Autodesk Inventor part; units mm, degrees
ref_plane "YZ Plane" through (0, 0, 0) normal (1, 0, 0) x (0, 1, 0)
ref_plane "XZ Plane" through (0, 0, 0) normal (0, 1, 0) x (-1, 0, 0)
ref_plane "XY Plane" through (0, 0, 0) normal (0, 0, 1) x (1, 0, 0)
sketch "Sketch1" plane through (0, 0, 0) normal (0, 1, 0) x (-1, 0, 0)
  line L0 (-97.5, -62.5) -> (97.5, -62.5)
  line L1 (97.5, 62.5) -> (-97.5, 62.5)
  line L2 (-97.5, 62.5) -> (-97.5, -62.5)
  line L3 (-97.5, -62.5) -> (97.5, 62.5) construction
  line L4 (97.5, -62.5) -> (-97.5, 62.5) construction
  line L5 (97.5, 20) -> (112.525, 20)
  line L6 (127.475, 21.2237) -> (127.475, -18.7763)
  line L7 (112.525, -17.5526) -> (97.5, -17.5526)
  line L8 (97.5, -62.5) -> (97.5, -17.5526)
  line L9 (97.5, 20) -> (97.5, 62.5)
  line L10 (112.525, 20) -> (112.525, 61)
  line L11 (127.475, 61) -> (127.475, 21.2237)
  line L12 (127.475, 1.2237) -> (97.475, 1.2237) construction
  line L13 (112.525, -17.5526) -> (112.525, -58.5526)
  line L14 (127.475, -58.5526) -> (127.475, -18.7763)
  line L15 (119.975, 61) -> (121.775, 61) construction
  line L16 (112.525, 61) -> (118.225, 61)
  line L17 (127.475, 61) -> (121.775, 61)
  line L18 (119.975, -58.5526) -> (121.775, -58.5526) construction
  line L19 (112.525, -58.5526) -> (118.225, -58.5526)
  line L20 (127.475, -58.5526) -> (121.775, -58.5526)
  line L21 (119.975, -58.5526) -> (121.775, -58.5526) construction
  line L22 (121.775, -58.5526) -> (121.775, -56.5526)
  line L23 (118.225, -58.5526) -> (118.225, -56.5526)
  line L24 (121.775, -56.5526) -> (125.775, -56.5526)
  line L25 (125.775, -56.5526) -> (125.775, -53.5526)
  line L26 (114.175, -53.5526) -> (118.175, -53.5526)
  line L27 (114.175, -56.5526) -> (114.175, -53.5526)
  line L28 (118.225, -56.5526) -> (114.175, -56.5526)
  line L29 (112.525, -58.5526) -> (118.225, -58.5526)
  line L30 (127.475, -58.5526) -> (121.775, -58.5526)
  line L31 (127.475, 61) -> (127.475, 79) construction
  line L32 (-97.5, 0) -> (-67.5, 0) construction
  line L33 (-67.5, 62.5) -> (-67.5, -62.5) construction
  line L34 (127.475, 79) -> (-67.5, 0) construction
  line L35 (127.475, -58.5526) -> (127.475, -76.5526) construction
  line L36 (127.475, -76.5526) -> (-67.5, 0) construction
  line L37 (-97.5, 62.5) -> (-117.5, 62.5)
  line L38 (-117.5, 62.5) -> (-117.5, -62.5)
  line L39 (-117.5, -62.5) -> (-97.5, -62.5)
  line L40 (-97.5, -62.5) -> (-97.5, 62.5)
  line L41 (-67.5, 0) -> (-47.5, 0) construction
  circle A0 centre (-47.5, 0) radius 1.6
  line L42 (-67.5, 0) -> (-87.5, 0) construction
  circle A1 centre (-87.5, 0) radius 1.6
  line L43 (121.775, 61) -> (118.225, 61)
  line L44 (125.775, -53.5526) -> (118.175, -53.5526)
  line L45 (121.775, -58.5526) -> (118.225, -58.5526)
  point P0 (0, 0)
  point P1 (-97.5, -62.5)
  dimension "d0" = 195
  dimension "d1" = 125
  dimension "d3" = 30
  dimension "d4" = 40
  dimension "d5" = 15
  dimension "d6" = 41
  dimension "d12" = 1.8
  dimension "d21" = 30
  dimension "d23" = 1.5
  dimension "d28" = 18
  dimension "d29" = 30
  dimension "d30" = 18
  dimension "d35" = 20
  dimension "d36" = 125
  dimension "d41" = 20
  dimension "d42" = 3.2
  dimension "d43" = 20
  dimension "d47" = 3.2
extrude "Extrusion1" add sketch "Sketch1" along normal blind 3.25 contours L2 L1 L9 L5 L10 L16 L43 L17 L11 L6 L14 L20 L22 L24 L25 L44 L26 L27 L28 L23 L19 L13 L7 L8 L0 | L23 L28 L27 L26 L44 L25 L24 L22 L45 | A0 | A1
sketch "Sketch2" plane through (0, 3.25, 0) normal (0, 1, 0) x (1, 0, 0)
  line L0 (-127.475, 58.5526) -> (-127.475, -61) construction
  line L1 (-127.475, 0) -> (-59.475, 0) construction
  circle A0 centre (-59.475, 0) radius 5
  point P0 (0, 0)
  dimension "d31" = 68
  dimension "d32" = 10
extrude "Extrusion2" cut sketch "Sketch2" against normal blind 10
sketch "Sketch3" plane through (97.5, 0, 62.5) normal (1, 0, 0) x (0, 0, -1)
  line L0 (125, 0) -> (80.0526, 0)
  line L1 (0, 3.25) -> (125, 3.25)
  line L2 (125, 3.25) -> (125, 0)
  line L3 (125, 0) -> (0, 0)
  line L4 (0, 0) -> (0, 3.25)
  point P0 (62.5, 0)
extrude "Extrusion4" add sketch "Sketch3" along normal blind 30
extrude "Extrusion5" cut sketch "Sketch1" along normal blind 4 contours A0 | A1
sketch "Sketch4" plane through (0, 3.25, 0) normal (0, 1, 0) x (1, 0, 0)
  line L0 (-97.5, -62.5) -> (127.5, -62.5) construction
  line L1 (39.3, -62.5) -> (39.3, -44.9) construction
  line L2 (127.5, 62.5) -> (127.5, -62.5) construction
  circle A0 centre (39.3, -44.9) radius 1.6
  circle A1 centre (16.42, -44.9) radius 1.6
  line L3 (39.3, -44.9) -> (16.42, -44.9) construction
  line L4 (118.8, -62.5) -> (118.8, -12.2) construction
  circle A2 centre (118.8, -12.2) radius 1.6
  line L5 (118.8, -12.2) -> (95.92, -12.2) construction
  circle A3 centre (95.92, -12.2) radius 1.6
  line L6 (-97.5, 62.5) -> (127.5, 62.5) construction
  line L7 (119.5, 62.5) -> (119.5, 35.9) construction
  circle A4 centre (119.5, 35.9) radius 1.6
  line L8 (119.5, 35.9) -> (96.62, 35.9) construction
  circle A5 centre (96.62, 35.9) radius 1.6
  line L9 (38.32, 62.5) -> (38.32, 33.4) construction
  circle A6 centre (38.32, 33.4) radius 1.6
  line L10 (38.32, 33.4) -> (15.44, 33.4) construction
  circle A7 centre (15.44, 33.4) radius 1.6
  point P0 (0, 0)
  point P1 (119.5, 49.2)
  dimension "d48" = 88.2
  dimension "d49" = 17.6
  dimension "d50" = 3.2
  dimension "d51" = 3.2
  dimension "d52" = 22.88
  dimension "d53" = 50.3
  dimension "d54" = 8.7
  dimension "d55" = 3.2
  dimension "d56" = 3.2
  dimension "d57" = 22.88
  dimension "d58" = 8
  dimension "d59" = 26.6
  dimension "d60" = 3.2
  dimension "d61" = 22.88
  dimension "d62" = 3.2
  dimension "d63" = 89.18
  dimension "d64" = 29.1
  dimension "d65" = 3.2
  dimension "d66" = 22.88
  dimension "d67" = 3.2
extrude "Extrusion6" cut sketch "Sketch4" against normal blind 10
sketch "Sketch5" plane through (0, 3.25, 0) normal (0, 1, 0) x (1, 0, 0)
  circle A0 centre (119.5, 35.9) radius 1.6 construction
  line L0 (123.5, 48.9829) -> (78.5, 48.9829) construction
  line L1 (123.5, 46.1029) -> (33.5, 46.1029)
  line L2 (33.5, 46.1029) -> (33.5, 51.8629)
  line L3 (33.5, 51.8629) -> (123.5, 51.8629)
  line L4 (123.5, 51.8629) -> (123.5, 46.1029)
  line L5 (123.5, 46.1029) -> (33.5, 51.8629) construction
  line L6 (33.5, 46.1029) -> (123.5, 51.8629) construction
  line L7 (127.5, 62.5) -> (127.5, -62.5)
  circle A1 centre (15.44, 33.4) radius 1.6 construction
  line L8 (11.5, 20.4) -> (56.5, 20.4) construction
  line L9 (101.5, 17.525) -> (11.5, 17.525)
  line L10 (11.5, 17.525) -> (11.5, 23.275)
  line L11 (11.5, 23.275) -> (101.5, 23.275)
  line L12 (101.5, 23.275) -> (101.5, 17.525)
  line L13 (101.5, 17.525) -> (11.5, 23.275) construction
  line L14 (11.5, 17.525) -> (101.5, 23.275) construction
  circle A2 centre (95.92, -12.2) radius 1.6 construction
  line L15 (111.5, -28.5) -> (66.5, -28.5) construction
  line L16 (124, -35.5) -> (9, -35.5)
  line L17 (9, -35.5) -> (9, -21.5)
  line L18 (9, -21.5) -> (124, -21.5)
  line L19 (124, -21.5) -> (124, -35.5)
  line L20 (124, -35.5) -> (9, -21.5) construction
  line L21 (9, -35.5) -> (124, -21.5) construction
  line L22 (-97.5, -62.5) -> (127.5, -62.5)
  point P0 (0, 0)
  dimension "d71" = 45
  dimension "d72" = 90
  dimension "d73" = 5.76
  dimension "d76" = 4
  dimension "d78" = 45
  dimension "d79" = 90
  dimension "d80" = 5.75
  dimension "d82" = 26
  dimension "d84" = 45
  dimension "d85" = 115
  dimension "d86" = 14
  dimension "d87" = 3.5
  dimension "d88" = 27
extrude "Extrusion7" cut sketch "Sketch5" against normal blind 10
sketch "Sketch8" plane through (0, 3.25, 0) normal (0, 1, 0) x (1, 0, 0)
  line L0 (-127.475, -61) -> (-112.525, -61) construction
  line L1 (-120, -61) -> (-121.75, -61) construction
  line L2 (-120, -61) -> (-118.25, -61) construction
  line L3 (-121.75, -61) -> (-121.75, -54)
  line L4 (-121.75, -54) -> (-123.95, -54)
  line L5 (-123.95, -54) -> (-123.95, -51.4)
  line L6 (-123.95, -51.4) -> (-121.75, -51.4)
  line L7 (-121.75, -51.4) -> (-121.75, -47)
  line L8 (-121.75, -47) -> (-118.25, -47)
  line L9 (-120, -61) -> (-120, -55.9834) construction
  line L10 (-118.25, -61) -> (-118.25, -54)
  line L11 (-118.25, -54) -> (-116.05, -54)
  line L12 (-116.05, -54) -> (-116.05, -51.4)
  line L13 (-116.05, -51.4) -> (-118.25, -51.4)
  line L14 (-118.25, -51.4) -> (-118.25, -47)
  line L15 (-127.475, 58.5526) -> (-127.475, -61) construction
  line L16 (-127.475, -1.2237) -> (-118.25, -1.2237) construction
  line L17 (-121.75, 58.5526) -> (-121.75, 51.5526)
  line L18 (-121.75, 51.5526) -> (-123.95, 51.5526)
  line L19 (-123.95, 51.5526) -> (-123.95, 48.9526)
  line L20 (-123.95, 48.9526) -> (-121.75, 48.9526)
  line L21 (-121.75, 48.9526) -> (-121.75, 44.5526)
  line L22 (-121.75, 44.5526) -> (-118.25, 44.5526)
  line L23 (-120, 58.5526) -> (-120, 53.536) construction
  line L24 (-118.25, 58.5526) -> (-118.25, 51.5526)
  line L25 (-118.25, 51.5526) -> (-116.05, 51.5526)
  line L26 (-116.05, 51.5526) -> (-116.05, 48.9526)
  line L27 (-116.05, 48.9526) -> (-118.25, 48.9526)
  line L28 (-118.25, 48.9526) -> (-118.25, 44.5526)
  line L29 (-121.75, -61) -> (-118.25, -61)
  line L30 (-121.75, 58.5526) -> (-118.25, 58.5526)
  line L31 (-112.525, 58.5526) -> (-127.475, 58.5526)
  point P0 (0, 0)
  dimension "d102" = 1.75
  dimension "d103" = 1.75
  dimension "d104" = 7
  dimension "d105" = 2.2
  dimension "d106" = 2.6
  dimension "d108" = 14
  dimension "d109" = 3.5
  dimension "d110" = 7
  dimension "d111" = 2.2
  dimension "d112" = 2.6
extrude "Extrusion10" cut sketch "Sketch8" against normal blind 3.25
properties part number "suelo_imp"
Read the model definition and answer for the solid it produces. Units are mm, in the model's axes. Give positions to 0.01 mm unless a question says otherwise; leave off trailing zeros. Write each loop counter-clockwise with the first axis right and the second up, starting at its lowest first coordinate (ties: lowest second). Pieces come first, ordered by that corner, then holes. Notation, with made-up numbers: (74, 76.25) - (114, 76.25) arc R13 ccw to (114, 91.25) - close; hole circle Ø5 at (76, 9.5). An arc over 180 degrees is marked (long way). Use CSV: the item, a comma, the result in double quotes. Start each with the question number.
Item 1: Flat-ended cylindrical pins translate along their axes: P1, Ø1.6, axis at x = -123.5, y = 2, coming from the -Z side; P2, Ø1.6, axis at x = -102.5, y = 2, coming from the +Z side. Find the tip coordinate at first contact, or state that the pin passes through.
Item 2: The part is cut by section A-A, the plane x = 83. Give the vertices of the cut face in (y, z) (3 decimals).
Item 3: The part is cut by section D-D, the plane y = 1.25. Count the separate pieces of the cut face and the enclosed holes in it, and give its area (3 significant figures).
Item 4: Consider line 1 (Z direction, x = 47.5, y = 1.6) (3 decimals); line 2 (X direction, y = 0.4, z = -22) (3 decimals); line 3 (X direction, y = 0.55, z = 55.5) (3 decimals). Determine where each line is inside the solid, lowest interval first.
Item 5: The part is cut by section C-C, the plane z = -21. Give the vertices of the cut face in (x, y) (3 decimals).
Item 6: The part is cut by section B-B, the plane z = 28.5. Give the vertices of the cut face in (x, y) (3 decimals), and give its area (3 significant figures).
Taken from the geometry:
1,P1,"z = -58.55"
1,P2,"z = 20"
2,outline,"(0, -62.5) - (3.25, -62.5) - (3.25, -51.863) - (0, -51.863) - close; (0, -46.103) - (3.25, -46.103) - (3.25, -23.275) - (0, -23.275) - close; (0, -17.525) - (3.25, -17.525) - (3.25, 21.5) - (0, 21.5) - close; (0, 35.5) - (3.25, 35.5) - (3.25, 62.5) - (0, 62.5) - close"
3,separate pieces,"1"
3,enclosed holes,"14"
3,area,"27,600 mm2"
4,line 1,"-62.5 to -51.863, -46.103 to -23.275, -17.525 to -1.6, 1.6 to 21.5, 35.5 to 62.5"
4,line 2,"-127.475 to -112.525, -97.5 to 11.5, 101.5 to 127.5"
4,line 3,"-127.475 to -121.75, -118.25 to -112.525, -97.5 to 127.5"
5,outline,"(-127.475, 0) - (-112.525, 0) - (-112.525, 3.25) - (-127.475, 3.25) - close; (-97.5, 0) - (11.5, 0) - (11.5, 3.25) - (-97.5, 3.25) - close; (101.5, 0) - (127.5, 0) - (127.5, 3.25) - (101.5, 3.25) - close"
6,outline,"(-127.475, 0) - (-112.525, 0) - (-112.525, 3.25) - (-127.475, 3.25) - close; (-97.5, 0) - (9, 0) - (9, 3.25) - (-97.5, 3.25) - close; (124, 0) - (127.5, 0) - (127.5, 3.25) - (124, 3.25) - close"
6,area,"406 mm2"
